from build123d import *

# Parameters (mm, degrees)
BASE_FLANGE1_DEPTH      = 70
FILLET1_R               = 10
SKETCH6_R               = 3.5
CUT_EXTRUDE1_DEPTH      = 10
EDGE_FLANGE2_DEPTH      = 40
EDGE_FLANGE2_START      = 2
EDGE_FLANGE2_FLAT_DEPTH = 2
SKETCH14_R              = 1.5
CUT_EXTRUDE2_DEPTH      = 10


# Sheet-metal steps are written as plain solids
with BuildPart() as part:
    # Sketch1 → Base-Flange1 (new body)
    with BuildSketch(Plane.XY):
        with BuildLine():
            Line((-65, 0), (-39, 0))
            ThreePointArc((-39, 0), (-36.171572875, 1.171572875), (-35, 4))
            Line((-35, 4), (-35, 68))
            ThreePointArc((-35, 68), (-34.414213562, 69.414213562), (-33, 70))
            Line((-33, 70), (33, 70))
            ThreePointArc((33, 70), (34.414213562, 69.414213562), (35, 68))
            Line((35, 68), (35, 4))
            ThreePointArc((35, 4), (36.171572875, 1.171572875), (39, 0))
            Line((39, 0), (65, 0))
            Line((65, 0), (65, 2))
            Line((65, 2), (39, 2))
            ThreePointArc((39, 2), (37.585786438, 2.585786438), (37, 4))
            Line((37, 4), (37, 68))
            ThreePointArc((37, 68), (35.828427125, 70.828427125), (33, 72))
            Line((33, 72), (-33, 72))
            ThreePointArc((-33, 72), (-35.828427125, 70.828427125), (-37, 68))
            Line((-37, 68), (-37, 4))
            ThreePointArc((-37, 4), (-37.585786438, 2.585786438), (-39, 2))
            Line((-39, 2), (-65, 2))
            Line((-65, 2), (-65, 0))
        make_face()
    extrude(amount=BASE_FLANGE1_DEPTH)

    # Fillet1
    fillet1_edges = [part.edges().sort_by_distance(p)[0] for p in [
        (65, 1, 0),
        (-65, 1, 0),
        (65, 1, 70),
        (-65, 1, 70),
    ]]
    fillet(fillet1_edges, radius=FILLET1_R)

    # Sketch6 → Cut-Extrude1 (cut)
    with BuildSketch(Plane(origin=(0, 2, 0), x_dir=(1, 0, 0), z_dir=(0, 1, 0))):
        with Locations(Location((-50, -15, 0), (0, 0, 180))):
            Circle(SKETCH6_R)
        with Locations(Location((-50, -55, 0), (0, 0, 180))):
            Circle(SKETCH6_R)
        with Locations((50, -55)):
            Circle(SKETCH6_R)
        with Locations((50, -15)):
            Circle(SKETCH6_R)
    extrude(amount=-CUT_EXTRUDE1_DEPTH, mode=Mode.SUBTRACT)

    # Edge-Flange2 bend section (across the edge) → Edge-Flange2 (add)
    with BuildSketch(Plane(origin=(-20, 72, 72), x_dir=(0, 0, -1), z_dir=(1, 0, 0))):
        with BuildLine():
            Line((-2, 2), (0, 2))
            ThreePointArc((0, 2), (0.585786438, 0.585786438), (2, 0))
            Line((2, 0), (2, -2))
            ThreePointArc((2, -2), (-0.828427125, -0.828427125), (-2, 2))
        make_face()
    extrude(amount=EDGE_FLANGE2_DEPTH)

    # Edge-Flange2 profile (on flange) → Edge-Flange2 flat (add)
    with BuildSketch(Plane(origin=(0, 72, 72), x_dir=(1, 0, 0), z_dir=(0, 0, 1)).offset(EDGE_FLANGE2_START)):
        with BuildLine():
            ThreePointArc((20, 22), (14.727922061, 34.727922061), (2, 40))
            Line((2, 40), (-2, 40))
            ThreePointArc((-2, 40), (-14.727922061, 34.727922061), (-20, 22))
            Line((-20, 22), (-20, 2))
            Line((-20, 2), (20, 2))
            Line((20, 2), (20, 22))
        make_face()
    extrude(amount=-EDGE_FLANGE2_FLAT_DEPTH)

    # Sketch14 → Cut-Extrude2 (cut)
    with BuildSketch(Plane.XY.offset(74)):
        with Locations((0, 106.30073689)):
            Circle(SKETCH14_R)
        with Locations((-12.817814143, 84.099631551)):
            Circle(SKETCH14_R)
        with Locations((12.817814144, 84.099631551)):
            Circle(SKETCH14_R)
        with BuildLine():
            ThreePointArc((0, 90.999999997), (-6.5, 84.499999998), (-1e-09, 77.999999997))
            ThreePointArc((-1e-09, 77.999999997), (6.5, 84.499999997), (0, 90.999999997))
        make_face()
    extrude(amount=-CUT_EXTRUDE2_DEPTH, mode=Mode.SUBTRACT)


solid = part.part
The listing builds one solid part. Answer for the finished solid, in the listing's coordinates (mm). A direction names the side the tool comes from. Coordinates: 2 decimals unless noted, no trailing zeros. Order: outer loops, then holes, each group sorted by start corner. A loop starts at its lowest first (then second) coordinate and runs counter-clockwise, first axis right, second up. Notation, with made-up numbers: M -40,44 L 1,44 A16 ccw 1,64 Z; hole C 26.5,83.5 d6. An arc over 180 degrees is marked long. Use CSV: the item, a comma, the result in double quotes.
Q1. A tool of negligible diameter and unlimited length cuts with its end or side. For faces 1 (the flat face through (37, 36, 35)), 2 (the cylindrical face through (-36.203, 1.141, 34.51)), 3 (the flat face through (36, 34, 70)), from which of +Z, -Z, +X, -X, +Y, -Y can it reach the whole face along a straight path? Write none if from no direction.
Here are the results:
face 1,"+Z, -Z, +X, +Y"
face 2,"+Z, -Z, -Y"
face 3,"+Z, +X, +Y, -Y"
Q2. Straight lines are drawn through the part: L1, parallel to Z at x = 50, y = 1; L2, parallel to X at y = 13, z = 37.5; L3, parallel to Y at x = 39, z = 50. For each, find the intervals that lie inside material, in ascending order.
Here are the results:
L1,"0 to 11.5, 18.5 to 51.5, 58.5 to 70"
L2,"-37 to -35, 35 to 37"
L3,"0 to 2"
Q3. Section C-C (x = 0) is taken. Determine the outline of the cut face in (y, z).
Here are the results:
outline,"M 70,0 L 72,0 L 72,70 A2 cw 74,72 L 78,72 L 78,74 L 74,74 A4 ccw 70,70 Z; M 91,72 L 104.8,72 L 104.8,74 L 91,74 Z; M 107.8,72 L 112,72 L 112,74 L 107.8,74 Z"
Q4. Given pin 1 Ø8 at (x, z) = (-50, 15) entering from +Y; pin 2 Ø1.5 at (x, z) = (-20.5, 66) entering from -Y; pin 3 Ø4 at (x, z) = (50, 15) entering from +Y; pin 4 Ø1.5 at (y, z) = (18, 22) entering from +X, each flat-ended and moving along its own axis, determine where each tip first touches the part or whether it passes through.
Here are the results:
pin 1,"y = 2"
pin 2,"y = 70"
pin 3,"through"
pin 4,"x = 37"
Q5. Section B-B (y = 14.5) is taken. Determine the outline of the cut face in (x, z), then the cut area to 3 significant figures.
Here are the results:
outline,"M -37,0 L -35,0 L -35,70 L -37,70 Z; M 35,0 L 37,0 L 37,70 L 35,70 Z"
area,"280 mm2"
Q6. Section A-A (z = 55) is taken. Determine the outline of the cut face in (x, y), then the cut area to 3 significant figures.
Here are the results:
outline,"M -65,0 L -53.5,0 L -53.5,2 L -65,2 Z; M -46.5,0 L -39,0 A4 ccw -35,4 L -35,68 A2 cw -33,70 L 33,70 A2 cw 35,68 L 35,4 A4 ccw 39,0 L 46.5,0 L 46.5,2 L 39,2 A2 cw 37,4 L 37,68 A4 ccw 33,72 L -33,72 A4 ccw -37,68 L -37,4 A2 cw -39,2 L -46.5,2 Z; M 53.5,0 L 65,0 L 65,2 L 53.5,2 Z"
area,"502 mm2"
Q7. Determine the mould class of faces 4 (the cylindrical face through (-62.15, 0.99, 3.01)), 5 (the cylindrical face through (-46.503, 1.014, 15.154)), 6 (the flat face through (52, 2, 35)) for opening direction X: pulls with the +X half, pulls with the -X half, needs draft (parallel to the pull), parting line crosses it, or undercut.
Here are the results:
face 4,"pulls with the -X half"
face 5,"undercut"
face 6,"needs draft"
Q8. Section D-D (x = -50) is taken. Determine the outline of the cut face in (y, z).
Here are the results:
outline,"M 0,0 L 2,0 L 2,11.5 L 0,11.5 Z; M 0,18.5 L 2,18.5 L 2,51.5 L 0,51.5 Z; M 0,58.5 L 2,58.5 L 2,70 L 0,70 Z"
